Source: CAD feature listing. Evaluate the final solid. Frame: model axes, mm. Face numbers are marked on the shaded views. Round coordinates to 2 decimals unless told otherwise and drop trailing zeros. Order: outer loops, then holes, each group sorted by start corner. A loop starts at its lowest first (then second) coordinate and runs counter-clockwise, first axis right, second up. Notation, with made-up numbers: (33, 63.25) -> (65, 63.25) arc R18 cw to (65, 70.25) -> close; hole circle Ø1 at (-2, 9). An arc over 180 degrees is marked (long way). One line per item, written item: value. Start each with the question number.
1) Section A-A (y = 18). Return the cut outline in (x, z).
2) Ray query, L1, parallel to Y at x = 19, z = -2; L2, parallel to Z at x = 10.5, y = 12; L3, parallel to Y at x = 22, z = 8. Return the intervals inside material, ascending.
3) Mould query, pull axis Y, two halves, no side actions, for the marked faces 1, 2, 3 and 4. Classes: pulls with the +Y half, pulls with the -Y half, needs draft (parallel to the pull), parting line crosses it, or undercut.
4) Pin query (flat end, axial travel): P1, Ø9, axis at y = 12, z = 0, coming from the +X side; P2, Ø4, axis at x = 4, y = 6.5, coming from the -Z side; P3, Ø10, axis at x = 8, y = 9.5, coming from the +Z side; P4, Ø1.5, axis at x = 18.5, y = 13.5, coming from the -Z side. Return the tip coordinate at first contact, or that it passes through.
```python
from build123d import *

# Parameters (mm, degrees)
SKETCH3_R               = 4
BOSS_EXTRUDE1_DEPTH     = 25
BOSS_EXTRUDE2_START     = 25
SKETCH3_5_R             = 3
BOSS_EXTRUDE2_DEPTH     = 8
CUT_EXTRUDE1_DEPTH      = 17
CUT_EXTRUDE1_DEPTH_BACK = 46.978255774
SKETCH15_R              = 1.8
FILLET3_R               = 1


with BuildPart() as part:
    # Sketch1 → Revolve1 (revolve)
    with BuildSketch(Plane.XY, mode=Mode.PRIVATE) as revolve1_sk:
        Polygon((0, 20), (0, 0), (25, 0), (25, 3), (23, 3), (23, 5), (10, 5), (10, 20), align=None)
    revolve(revolve1_sk.sketch.rotate(Axis((0, 20, 0), (0, -1, 0)), 90), axis=Axis((0, 20, 0), (0, -1, 0)))

    # Sketch3 → Boss-Extrude1 (add)
    with BuildSketch(Plane(origin=(0, 0, 0), x_dir=(0, 0, -1), z_dir=(1, 0, 0))):
        with Locations(Location((0, 12, 0), (0, 0, 180))):
            Circle(SKETCH3_R)
    extrude(amount=BOSS_EXTRUDE1_DEPTH)

    # Sketch3<5> → Boss-Extrude2 (add)
    with BuildSketch(Plane(origin=(0, 0, 0), x_dir=(0, 0, -1), z_dir=(1, 0, 0)).offset(BOSS_EXTRUDE2_START)):
        with Locations((0, 12)):
            Circle(SKETCH3_5_R)
    extrude(amount=BOSS_EXTRUDE2_DEPTH)

    # Sketch11 → Cut-Revolve10 (revolve, cut)
    with BuildSketch(Plane.XY):
        with BuildLine():
            Line((0, 4), (0, 0))
            Line((0, 0), (22.072872435, 0))
            ThreePointArc((22.072872435, 0), (11.216213299, 2.992049146), (0, 4))
        make_face()
    revolve(axis=Axis((0, 0, 0), (0, 1, 0)), mode=Mode.SUBTRACT)

    # Sketch15 → Cut-Extrude1 (cut, two sides: drawn at the far end of the back side and taken through both)
    with BuildSketch(Plane(origin=(0, 0, 0), x_dir=(1, 0, 0), z_dir=(0, 1, 0)).offset(-CUT_EXTRUDE1_DEPTH_BACK)):
        with Locations(Location((0, 0, 0), (0, 0, 270))):
            Circle(SKETCH15_R)
    extrude(amount=CUT_EXTRUDE1_DEPTH + CUT_EXTRUDE1_DEPTH_BACK, mode=Mode.SUBTRACT)

    # Sketch16 → Cut-Revolve12 (revolve, cut)
    with BuildSketch(Plane.XY, mode=Mode.PRIVATE) as cut_revolve12_sk:
        Polygon((33, 15), (33, 13.5), (15.503373698, 16), (33, 16), align=None)
    revolve(cut_revolve12_sk.sketch.rotate(Axis((33, 12, 0), (-1, 0, 0)), 270), axis=Axis((33, 12, 0), (-1, 0, 0)), mode=Mode.SUBTRACT)

    # Sketch17 → Cut-Revolve13 (revolve, cut)
    with BuildSketch(Plane.XY, mode=Mode.PRIVATE) as cut_revolve13_sk:
        Polygon((33, 12.6), (33, 12), (0, 12), (0, 14.8), (15.503373698, 14.8), (30.900404844, 12.6), align=None)
    revolve(cut_revolve13_sk.sketch.rotate(Axis((33, 12, 0), (-1, 0, 0)), 90), axis=Axis((33, 12, 0), (-1, 0, 0)), mode=Mode.SUBTRACT)

    # Fillet3
    fillet3_edges = [part.edges().sort_by_distance(p)[0] for p in [
        (9.16515139, 12, -4),
        (15.503373698, 12, -4),
        (33, 12, -1.5),
    ]]
    fillet(fillet3_edges, radius=FILLET3_R)


solid = part.part
```
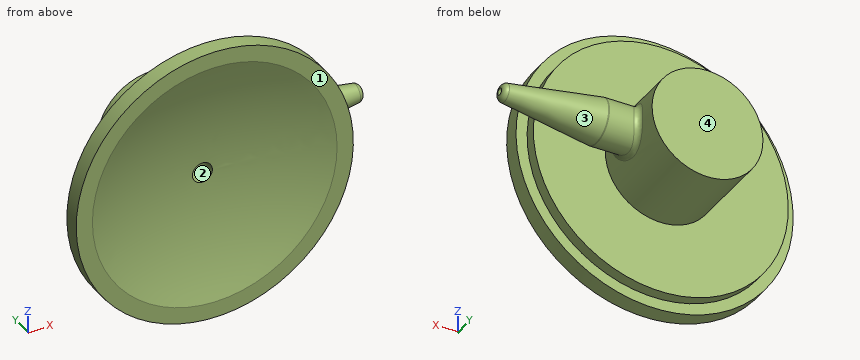
Findings:
1. outline: circle Ø20 at (0, 0)
2. L1: 1.03 to 5, 9.13 to 10.86, 13.14 to 14.87
2. L2: -4 to -2.8, 2.8 to 4
2. L3: 0 to 3
3. face 1: pulls with the -Y half
3. face 2: needs draft
3. face 3: undercut
3. face 4: pulls with the +Y half
4. P1: x = 33
4. P2: z = -22.84
4. P3: z = 22.25
4. P4: z = -3.52
